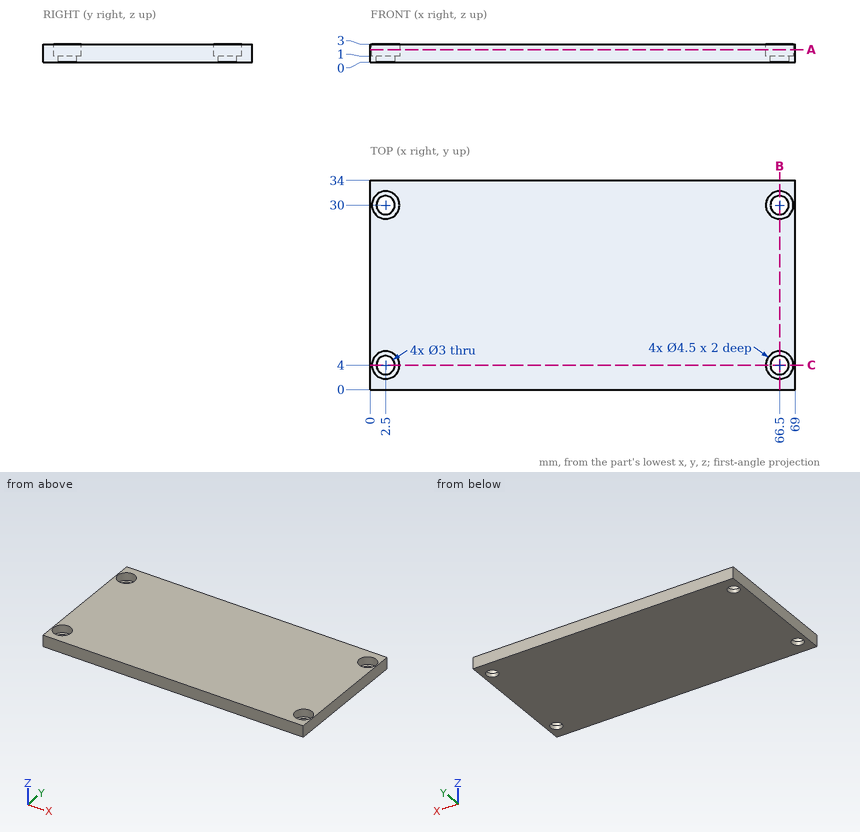
Can you work these out from the drawing? Everything is in mm from the part's minimum corner. Give positions to 0.01 mm unless a question says otherwise; leave off trailing zeros. Loops run counter-clockwise (first coordinate to the right, second up) from the corner with the lowest first, then second, coordinate; pieces in that order, holes last. Notation, with made-up numbers: (58.5, -36) - (94.5, -36) arc R20 cw to (94.5, -31) - close; hole circle Ø4 at (-7, 45). An arc over 180 degrees is marked (long way). Answer as a JSON object with one key per item and string values.
Q1. Imagine slicing it at B-B on x = 66.5. Write out the boundary of the cut face in (y, z).
Geometry says:
{"outline": "(0, 0) - (2.5, 0) - (2.5, 1) - (1.75, 1) - (1.75, 3) - (0, 3) - close; (5.5, 0) - (28.5, 0) - (28.5, 1) - (27.75, 1) - (27.75, 3) - (6.25, 3) - (6.25, 1) - (5.5, 1) - close; (31.5, 0) - (34, 0) - (34, 3) - (32.25, 3) - (32.25, 1) - (31.5, 1) - close"}
Q2. Will this pin go through, and if not, where does the flat tip stop? P1, Ø2, axis at x = 67, y = 29.5, coming from the +Z side.
Geometry says:
{"P1": "z = 1"}
Q3. Imagine slicing it at C-C on y = 4. Write out the boundary of the cut face in (x, z), plus the area to 3 significant figures.
Geometry says:
{"outline": "(0, 0) - (1, 0) - (1, 1) - (0.25, 1) - (0.25, 3) - (0, 3) - close; (4, 0) - (65, 0) - (65, 1) - (64.25, 1) - (64.25, 3) - (4.75, 3) - (4.75, 1) - (4, 1) - close; (68, 0) - (69, 0) - (69, 3) - (68.75, 3) - (68.75, 1) - (68, 1) - close", "area": "183 mm²"}
Q4. Imagine slicing it at A-A on z = 2.1. Write out the boundary of the cut face in (x, y).
Geometry says:
{"outline": "(0, 0) - (69, 0) - (69, 34) - (0, 34) - close; hole circle Ø4.5 at (2.5, 4); hole circle Ø4.5 at (2.5, 30); hole circle Ø4.5 at (66.5, 4); hole circle Ø4.5 at (66.5, 30)"}
Q5. If I drill on L1, parallel to Y at x = 2.5, z = 0.8; L2, parallel to Y at x = 2.5, z = 2.3; L3, parallel to X at y = 3.5, z = 1.3, over which ranges is the centre line in solid material (lowest first)?
Geometry says:
{"L1": "0 to 2.5, 5.5 to 28.5, 31.5 to 34", "L2": "0 to 1.75, 6.25 to 27.75, 32.25 to 34", "L3": "0 to 0.31, 4.69 to 64.31, 68.69 to 69"}
